Check sheet for the modelled part. Datum: model origin and axes. Units: mm. Round coordinates to 2 decimals unless told otherwise and drop trailing zeros. Write each loop counter-clockwise with the first axis right and the second up, starting at its lowest first coordinate (ties: lowest second). Pieces come first, ordered by that corner, then holes.
Item 1: Cross-section at A-A on x = 267. Enter the section's corners in (y, z).
Item 2: Release check for a two-part mould opening along X. For faces 1 (the flat face through (236, 0, -162)), 2 (the cylindrical face through (58.764, 1.521, -40.994)) record: +X half, -X half, draft (parallel to the pull), parting line (faces both ways), or undercut.
Item 3: Cross-section at B-B on y = 2.3. Enter the section's corners in (x, z), plus the area to 3 significant figures.
Item 4: Go/stop test with a flat-tipped pin: pin 1 Ø3.5 at (x, z) = (349, -200) entering from +Y. Record where the tip stops, or that it passes through.
Item 5: Cross-section at C-C on z = -245. Enter the section's corners in (x, y), plus the area to 3 significant figures.
Item 6: Material ranges on line 1 (X direction, y = 1.25, z = -285); line 2 (Z direction, x = 349, y = 1.55); line 3 (X direction, y = 1.95, z = -36), recorded low to high.
Item 7: Cross-section at D-D on x = 164. Enter the section's corners in (y, z).
from build123d import *

# Parameters (mm, degrees)
ESQUISSE1_W             = 390
ESQUISSE1_H             = 320
BASE_EXTRUSION_DEPTH    = 3
ESQUISSE2_W             = 75
ESQUISSE2_H             = 200
ENL_V_MAT_EXTRU_1_DEPTH = 4
ESQUISSE3_R             = 6
ENL_V_MAT_EXTRU_2_DEPTH = 4
ESQUISSE4_R             = 3
ENL_V_MAT_EXTRU_3_DEPTH = 10


with BuildPart() as part:
    # Esquisse1 → Base-Extrusion (new body)
    with BuildSketch(Plane(origin=(0, 0, 0), x_dir=(1, 0, 0), z_dir=(0, 1, 0))):
        with Locations((195, 160)):
            Rectangle(ESQUISSE1_W, ESQUISSE1_H)
    extrude(amount=BASE_EXTRUSION_DEPTH)

    # Esquisse2 → Enlèv. mat.-Extru.1 (cut)
    with BuildSketch(Plane(origin=(0, 3, 0), x_dir=(-1, 0, 0), z_dir=(0, 1, 0))):
        with Locations((-172.5, -160)):
            Rectangle(ESQUISSE2_W, ESQUISSE2_H)
    extrude(amount=-ENL_V_MAT_EXTRU_1_DEPTH, mode=Mode.SUBTRACT)

    # Esquisse3 → Enlèv. mat.-Extru.2 (cut)
    with BuildSketch(Plane(origin=(0, 3, 0), x_dir=(-1, 0, 0), z_dir=(0, 1, 0))):
        with Locations(Location((-267, -285, 0), (0, 0, 90))):
            Circle(ESQUISSE3_R)
        with Locations(Location((-58.5, -285, 0), (0, 0, 90))):
            Circle(ESQUISSE3_R)
        with Locations(Location((-267, -35, 0), (0, 0, 90))):
            Circle(ESQUISSE3_R)
        with Locations(Location((-58.5, -35, 0), (0, 0, 90))):
            Circle(ESQUISSE3_R)
    extrude(amount=-ENL_V_MAT_EXTRU_2_DEPTH, mode=Mode.SUBTRACT)

    # Esquisse4 → Enlèv. mat.-Extru.3 (cut)
    with BuildSketch(Plane(origin=(0, 3, 0), x_dir=(-1, 0, 0), z_dir=(0, 1, 0))):
        with Locations(Location((-349, -200, 0), (0, 0, 90))):
            Circle(ESQUISSE4_R)
        with Locations(Location((-349, -120, 0), (0, 0, 90))):
            Circle(ESQUISSE4_R)
    extrude(amount=-ENL_V_MAT_EXTRU_3_DEPTH, mode=Mode.SUBTRACT)


solid = part.part
Response values:
1. outline: (0, -320) - (3, -320) - (3, -291) - (0, -291) - close; (0, -279) - (3, -279) - (3, -41) - (0, -41) - close; (0, -29) - (3, -29) - (3, 0) - (0, 0) - close
2. face 1: draft
2. face 2: undercut
3. outline: (0, -320) - (390, -320) - (390, 0) - (0, 0) - close; hole circle Ø12 at (58.5, -285); hole circle Ø12 at (58.5, -35); hole (135, -260) - (210, -260) - (210, -60) - (135, -60) - close; hole circle Ø12 at (267, -285); hole circle Ø12 at (267, -35); hole circle Ø6 at (349, -200); hole circle Ø6 at (349, -120)
3. area: 109,000 mm2
4. pin 1: passes through
5. outline: (0, 0) - (135, 0) - (135, 3) - (0, 3) - close; (210, 0) - (390, 0) - (390, 3) - (210, 3) - close
5. area: 945 mm2
6. line 1: x = 0 to 52.5, 64.5 to 261, 273 to 390
6. line 2: z = -320 to -203, -197 to -123, -117 to 0
6. line 3: x = 0 to 52.58, 64.42 to 261.08, 272.92 to 390
7. outline: (0, -320) - (3, -320) - (3, -260) - (0, -260) - close; (0, -60) - (3, -60) - (3, 0) - (0, 0) - close
